Model file for the job. Use its own axes, mm. A direction names the side the tool comes from. Give positions to 0.01 mm unless a question says otherwise; leave off trailing zeros. Write each loop counter-clockwise with the first axis right and the second up, starting at its lowest first coordinate (ties: lowest second). Pieces come first, ordered by that corner, then holes.
```python
from build123d import *

# Parameters (mm, degrees)
SKETCH1_W              = 152.672175124
SKETCH1_H              = 75.20671235
BASE_FLANGE1_DEPTH     = 2.54
SKETCHED_START         = -37.603356175
SKETCHED_BEND1_DEPTH   = 75.20671235
SKETCHED_BEND1_2_DEPTH = 75.20671235


# Read off the part's stored shape, not the designer's step: Sketched Bend1
# Sheet-metal steps are written as plain solids
with BuildPart() as part:
    # Sketch1 → Base-Flange1 (new body)
    with BuildSketch(Plane.XY):
        Rectangle(SKETCH1_W, SKETCH1_H)
    extrude(amount=-BASE_FLANGE1_DEPTH)

    # Sketched Bend1 outline → Sketched Bend1 (cut)
    with BuildSketch(Plane(origin=(0, 0, 0), x_dir=(1, 0, 0), z_dir=(0, 1, 0)).offset(SKETCHED_START)):
        with BuildLine():
            ThreePointArc((-39.8528381, 0), (-38.700029664, 1.827542266), (-36.660107607, 2.54))
            Line((-36.660107607, 2.54), (-76.336087562, 2.54))
            Line((-76.336087562, 2.54), (-76.336087562, 0))
            Line((-76.336087562, 0), (-39.8528381, 0))
        make_face()
        with BuildLine():
            Line((76.336087562, 2.54), (36.660107607, 2.54))
            ThreePointArc((36.660107607, 2.54), (38.700029664, 1.827542266), (39.8528381, 0))
            Line((39.8528381, 0), (76.336087562, 0))
            Line((76.336087562, 0), (76.336087562, 2.54))
        make_face()
    extrude(amount=SKETCHED_BEND1_DEPTH, mode=Mode.SUBTRACT)

    # Sketched Bend1 2 outline → Sketched Bend1 2 (add)
    with BuildSketch(Plane(origin=(0, 0, 0), x_dir=(1, 0, 0), z_dir=(0, 1, 0)).offset(SKETCHED_START)):
        with BuildLine():
            Line((-36.660107607, 0), (-39.8528381, 0))
            ThreePointArc((-39.8528381, 0), (-39.915672711, -0.365920336), (-39.936707607, -0.7366))
            Line((-39.936707607, -0.7366), (-39.936707607, -37.260620045))
            Line((-39.936707607, -37.260620045), (-37.396707607, -37.260620045))
            Line((-37.396707607, -37.260620045), (-37.396707607, -0.7366))
            ThreePointArc((-37.396707607, -0.7366), (-37.180962462, -0.215745145), (-36.660107607, 0))
        make_face()
        with BuildLine():
            ThreePointArc((39.936707607, -0.7366), (39.915672711, -0.365920336), (39.8528381, 0))
            Line((39.8528381, 0), (36.660107607, 0))
            ThreePointArc((36.660107607, 0), (37.180962462, -0.215745145), (37.396707607, -0.7366))
            Line((37.396707607, -0.7366), (37.396707607, -37.260620045))
            Line((37.396707607, -37.260620045), (39.936707607, -37.260620045))
            Line((39.936707607, -37.260620045), (39.936707607, -0.7366))
        make_face()
    extrude(amount=SKETCHED_BEND1_2_DEPTH)


solid = part.part
```
1. Probe probe 1 along X at (y, z) = (-10.5, 32); probe 2 along Z at (x, y) = (-2, 18). List the from-to ranges inside material, lowest first.
Calculated:
probe 1: x = -39.94 to -37.4, 37.4 to 39.94
probe 2: z = -2.54 to 0
2. Slice it at C-C, the plane x = 22. Write the cut outline in (y, z), and give its area (3 significant figures).
Calculated:
outline: (-37.6, -2.54) - (37.6, -2.54) - (37.6, 0) - (-37.6, 0) - close
area: 191 mm2
3. Slice it at B-B, the plane y = -31.5. Write the cut outline in (x, z), and give its area (3 significant figures).
Calculated:
outline: (-39.94, 0.74) arc R3.28 ccw to (-36.66, -2.54) - (36.66, -2.54) arc R3.28 ccw to (39.94, 0.74) - (39.94, 37.26) - (37.4, 37.26) - (37.4, 0.74) arc R0.74 cw to (36.66, 0) - (-36.66, 0) arc R0.74 cw to (-37.4, 0.74) - (-37.4, 37.26) - (-39.94, 37.26) - close
area: 388 mm2
4. Which spindle directions (+Z, -Z, +X, -X, +Y, -Y) get a long thin tool onto all of the face, cutting with end or side? Do faces 4 (the flat face through (-39.937, -1, 19)), 5 (the flat face through (37.397, -1, 19)). Say none if no direction does.
Calculated:
face 4: +Z, -Z, -X, +Y, -Y
face 5: +Z, +Y, -Y
5. Slice it at A-A, the plane z = 12.5. Write the cut outline in (x, y), and give its area (3 significant figures).
Calculated:
outline: (-39.94, -37.6) - (-37.4, -37.6) - (-37.4, 37.6) - (-39.94, 37.6) - close; (37.4, -37.6) - (39.94, -37.6) - (39.94, 37.6) - (37.4, 37.6) - close
area: 382 mm2
6. Pull direction X, two halves, no side cores. Call faces 1 (the flat face through (-1, 1, -2.54)), 2 (the flat face through (-1, 1, 0)), 3 (the flat face through (39.937, -1, 19)): +X half, -X half, draft (parallel to the pull), parting line (faces both ways), or undercut.
Calculated:
face 1: draft
face 2: undercut
face 3: +X half
